from build123d import *

# Parameters (mm, degrees)
CROQUIS1_R              = 11.05
SALIENTE_EXTRUIR1_DEPTH = 5.5
CHAFL_N1_SIZE           = 2
CHAFL_N1_SIZE2          = 0.7
CROQUIS2_R              = 9.35
CORTAR_EXTRUIR1_DEPTH   = 1.45
CROQUIS3_R              = 9.65
CORTAR_EXTRUIR2_DEPTH   = 3.1
CROQUIS4_R              = 2.45
CORTAR_EXTRUIR3_DEPTH   = 0.95
CROQUIS5_R              = 2.94693617
CORTAR_EXTRUIR4_DEPTH   = 7


with BuildPart() as part:
    # Croquis1 → Saliente-Extruir1 (new body)
    with BuildSketch(Plane(origin=(0, 0, 0), x_dir=(1, 0, 0), z_dir=(0, 1, 0))):
        with Locations(Location((0, 0, 0), (0, 0, 270))):
            Circle(CROQUIS1_R)
    extrude(amount=SALIENTE_EXTRUIR1_DEPTH)

    # Chaflán1
    chafl_n1_edges = [part.edges().sort_by_distance(p)[0] for p in [
        (0, 5.5, -11.05),
    ]]
    chafl_n1_side = [part.faces().sort_by_distance(p)[0] for p in [
        (0, 2.75, -11.05),
    ]]
    chamfer(chafl_n1_edges, length=CHAFL_N1_SIZE, length2=CHAFL_N1_SIZE2, reference=chafl_n1_side[0])

    # Croquis2 → Cortar-Extruir1 (cut)
    with BuildSketch(Plane(origin=(0, 5.5, 0), x_dir=(1, 0, 0), z_dir=(0, 1, 0))):
        with Locations(Location((0, 0, 0), (0, 0, 270))):
            Circle(CROQUIS2_R)
    extrude(amount=-CORTAR_EXTRUIR1_DEPTH, mode=Mode.SUBTRACT)

    # Croquis3 → Cortar-Extruir2 (cut)
    with BuildSketch(Plane.XZ):
        with Locations(Location((0, 0, 0), (0, 0, 270))):
            Circle(CROQUIS3_R)
    extrude(amount=-CORTAR_EXTRUIR2_DEPTH, mode=Mode.SUBTRACT)

    # Croquis4 → Cortar-Extruir3 (cut)
    with BuildSketch(Plane(origin=(0, 4.05, 0), x_dir=(1, 0, 0), z_dir=(0, 1, 0))):
        with Locations(Location((0, 0, 0), (0, 0, 270))):
            Circle(CROQUIS4_R)
        with Locations(Location((5.6, 0, 0), (0, 0, 270))):
            Circle(CROQUIS4_R)
        with Locations(Location((2.8, 4.849742261, 0), (0, 0, 270))):
            Circle(CROQUIS4_R)
        with Locations(Location((-2.8, 4.849742261, 0), (0, 0, 270))):
            Circle(CROQUIS4_R)
        with Locations(Location((-5.6, 0, 0), (0, 0, 270))):
            Circle(CROQUIS4_R)
        with Locations(Location((-2.8, -4.849742261, 0), (0, 0, 270))):
            Circle(CROQUIS4_R)
        with Locations(Location((2.8, -4.849742261, 0), (0, 0, 270))):
            Circle(CROQUIS4_R)
    extrude(amount=-CORTAR_EXTRUIR3_DEPTH, mode=Mode.SUBTRACT)

    # Croquis5 → Cortar-Extruir4 (cut)
    with BuildSketch(Plane.XZ):
        with Locations((5.107651345, 12.330961149)):
            Circle(CROQUIS5_R)
        with Locations((12.330961149, 5.107651345)):
            Circle(CROQUIS5_R)
        with Locations((12.330961149, -5.107651345)):
            Circle(CROQUIS5_R)
        with Locations((5.107651345, -12.330961149)):
            Circle(CROQUIS5_R)
        with Locations((-5.107651345, -12.330961149)):
            Circle(CROQUIS5_R)
        with Locations((-12.330961149, -5.107651345)):
            Circle(CROQUIS5_R)
        with Locations((-12.330961149, 5.107651345)):
            Circle(CROQUIS5_R)
        with Locations((-5.107651345, 12.330961149)):
            Circle(CROQUIS5_R)
    extrude(amount=-CORTAR_EXTRUIR4_DEPTH, mode=Mode.SUBTRACT)


solid = part.part
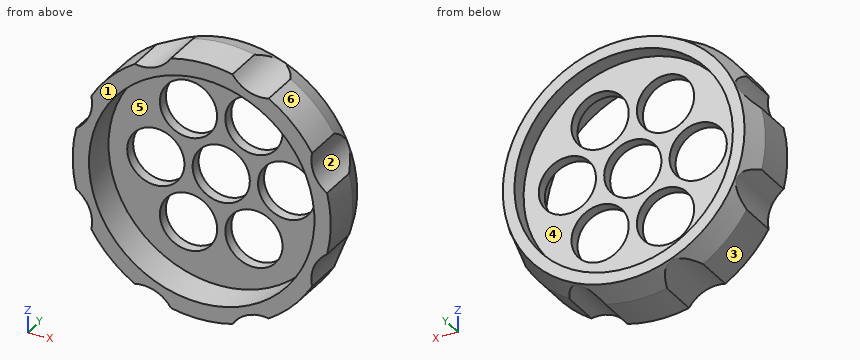
Here's how the part is built. I have some questions about the finished solid (model axes, mm). Face numbers are marked on the shaded views. A direction names the side the tool comes from. Coordinates: 2 decimals unless noted, no trailing zeros. Write each loop counter-clockwise with the first axis right and the second up, starting at its lowest first coordinate (ties: lowest second). Pieces come first, ordered by that corner, then holes.
Item 1: I want a section at B-B on y = 1.2. Write out the boundary of the cut face in (x, z), and give its area (3 significant figures).
Item 2: I want a section at A-A on z = 0. Write out the boundary of the cut face in (x, y).
Item 3: I want a section at D-D on x = -4.25. Count the separate pieces of the cut face and the enclosed holes in it, and give its area (3 significant figures).
Item 4: If we mould it in two halves opening along X, with no side actions, what happens to the marked faces 1, 2, 3 and 4? For each: +X half, -X half, draft (parallel to the pull), parting line (faces both ways), or undercut.
Item 5: On a 3-axis mill with a long thin cutter (end or side, diameter ignored), from which of +Z, -Z, +X, -X, +Y, -Y can I reach the whole of each face in a straight line? I mean the marked faces 5 and 6. Say none if no direction works.
Item 6: Will these pins go through, and if not, where does the flat tip stop? pin 1 (1.5 mm diameter, centred on y = 3.5, z = 5.5, fed in from +X); pin 2 (5.5 mm diameter, centred on x = -2.8, z = 4.85, fed in from +Y); pin 3 (1.5 mm diameter, centred on y = 2, z = 8.5, fed in from -X).
Item 7: I want a section at C-C on x = 0. Write out the boundary of the cut face in (y, z), and give its area (4 significant figures).
Item 8: If I drill on line 1 (X direction, y = 3.35, z = 0); line 2 (X direction, y = 3.5, z = 4); line 3 (Y direction, x = -3.5, z = 7.25), over which ranges is the centre line in solid material (lowest first)?
Findings below:
1. outline: (-10.73, -2.63) arc R2.95 cw to (-9.45, -5.73) arc R11.05 ccw to (-5.73, -9.45) arc R2.95 cw to (-2.63, -10.73) arc R11.05 ccw to (2.63, -10.73) arc R2.95 cw to (5.73, -9.45) arc R11.05 ccw to (9.45, -5.73) arc R2.95 cw to (10.73, -2.63) arc R11.05 ccw to (10.73, 2.63) arc R2.95 cw to (9.45, 5.73) arc R11.05 ccw to (5.73, 9.45) arc R2.95 cw to (2.63, 10.73) arc R11.05 ccw to (-2.63, 10.73) arc R2.95 cw to (-5.73, 9.45) arc R11.05 ccw to (-9.45, 5.73) arc R2.95 cw to (-10.73, 2.63) arc R11.05 ccw to start; hole circle Ø19.3 at (0, 0)
1. area: 79.2 mm2
2. outline: (-11.05, 0) - (-9.65, 0) - (-9.65, 3.1) - (-8.05, 3.1) - (-8.05, 4.05) - (-9.35, 4.05) - (-9.35, 5.5) - (-10.35, 5.5) - (-11.05, 3.5) - close; (-3.15, 3.1) - (-2.45, 3.1) - (-2.45, 4.05) - (-3.15, 4.05) - close; (2.45, 3.1) - (3.15, 3.1) - (3.15, 4.05) - (2.45, 4.05) - close; (8.05, 3.1) - (9.65, 3.1) - (9.65, 0) - (11.05, 0) - (11.05, 3.5) - (10.35, 5.5) - (9.35, 5.5) - (9.35, 4.05) - (8.05, 4.05) - close
3. separate pieces: 4
3. enclosed holes: 0
3. area: 15.4 mm2
4. face 1: draft
4. face 2: +X half
4. face 3: -X half
4. face 4: undercut
5. face 5: -Y
5. face 6: +Z, +X, +Y, -Y
6. pin 1: stops at x = 9.45
6. pin 2: stops at y = 4.05
6. pin 3: stops at x = -7.88
7. outline: (0, -11.05) - (3.5, -11.05) - (5.5, -10.35) - (5.5, -9.35) - (4.05, -9.35) - (4.05, -2.45) - (3.1, -2.45) - (3.1, -9.65) - (0, -9.65) - close; (0, 9.65) - (3.1, 9.65) - (3.1, 2.45) - (4.05, 2.45) - (4.05, 9.35) - (5.5, 9.35) - (5.5, 10.35) - (3.5, 11.05) - (0, 11.05) - close
7. area: 28.55 mm2
8. line 1: x = -11.05 to -8.05, -3.15 to -2.45, 2.45 to 3.15, 8.05 to 11.05
8. line 2: x = -9.6 to -5.1, -0.5 to 0.5, 5.1 to 9.6
8. line 3: y = 3.1 to 4.05
